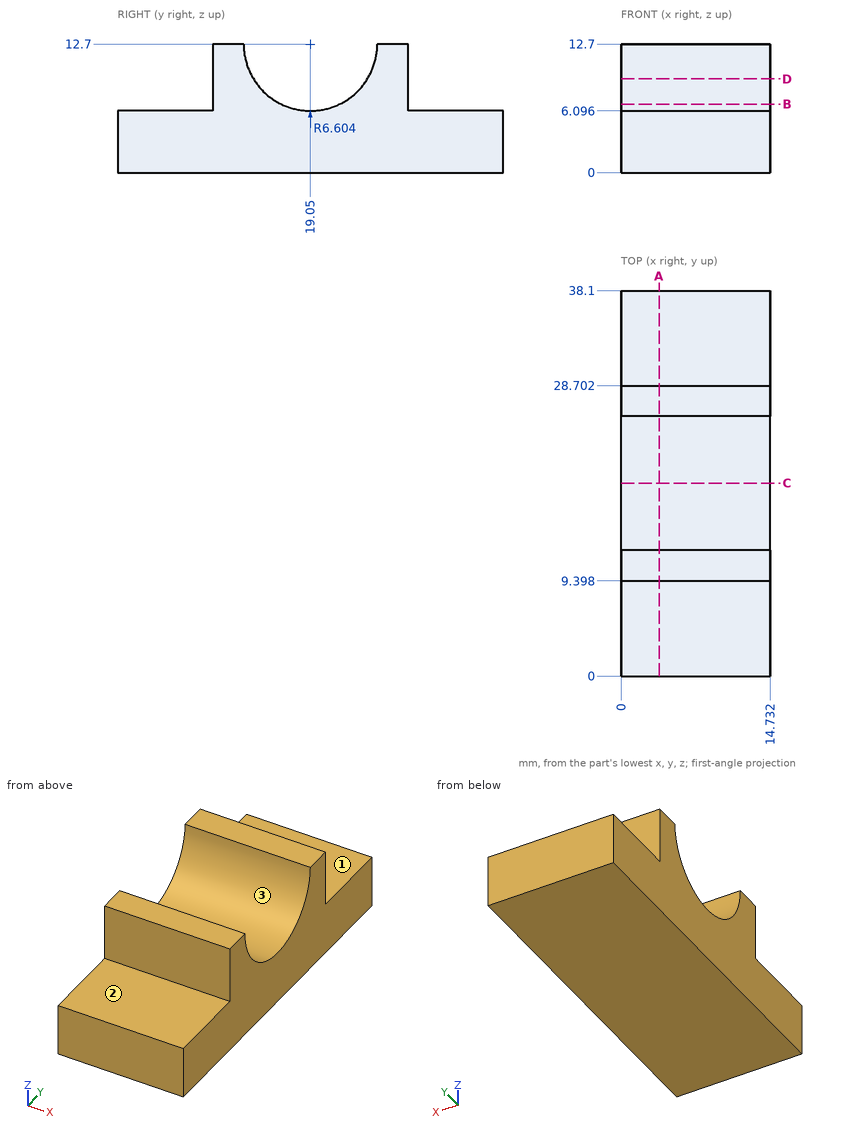
Geometry check sheet. Reference: drawing and pictorial views, mm from the part's lowest x, y, z. A direction names the side the tool comes from. Coordinates: 2 decimals unless noted, no trailing zeros. Order: outer loops, then holes, each group sorted by start corner. A loop starts at its lowest first (then second) coordinate and runs counter-clockwise, first axis right, second up. Notation, with made-up numbers: M 51,-26.5 L 56,-26.5 A24 ccw 56,-16.5 Z; hole C 34,-19 d9. An arc over 180 degrees is marked long. Return JSON: item names as keys, results as strings.
1) Access from +Z, -Z, +X, -X, +Y, -Y to the whole of each face (thin tool, end or side, straight path). Record for the marked faces 1, 2 and 3.
Answer list:
{"face 1": "+Z, +X, -X, +Y", "face 2": "+Z, +X, -X, -Y", "face 3": "+Z, +X, -X"}
2) Thickness scan on L1, parallel to Z at x = 13.5, y = 8; L2, parallel to Y at x = 9.75, z = 9.25; L3, parallel to Y at x = 13.25, z = 11.75. Record the ranges inside material, lowest first. Write a range as [from, to].
Answer list:
{"L1": "[0, 6.1]", "L2": "[9.4, 13.42], [24.68, 28.7]", "L3": "[9.4, 12.51], [25.59, 28.7]"}
3) Cross-section at D-D, the plane z = 9.25. Record the boundary of the cut face in (x, y).
Answer list:
{"outline": "M 0,9.4 L 14.73,9.4 L 14.73,13.42 L 0,13.42 Z; M 0,24.68 L 14.73,24.68 L 14.73,28.7 L 0,28.7 Z"}
4) Cross-section at A-A, the plane x = 3.75. Record the boundary of the cut face in (y, z), and give its area (3 significant figures).
Answer list:
{"outline": "M 0,0 L 38.1,0 L 38.1,6.1 L 28.7,6.1 L 28.7,12.7 L 25.65,12.7 A6.6 cw 12.45,12.7 L 9.4,12.7 L 9.4,6.1 L 0,6.1 Z", "area": "291 mm2"}
5) Cross-section at C-C, the plane y = 19.05. Record the boundary of the cut face in (x, z).
Answer list:
{"outline": "M 0,0 L 14.73,0 L 14.73,6.1 L 0,6.1 Z"}
6) Gauge pin test, flat ends, axial feed: pin 1 (3.5 mm diameter, centred on x = 5.5, z = 10, fed in from +Y); pin 2 (5 mm diameter, centred on x = 9, z = 5.5, fed in from -Y); pin 3 (5.5 mm diameter, centred on x = 7, z = 10.5, fed in from -Y); pin 4 (4.5 mm diameter, centred on x = 4.5, y = 35, fed in from +Z). Record the tip position at first contact, or that the pin passes through.
Answer list:
{"pin 1": "y = 28.7", "pin 2": "y = 0", "pin 3": "y = 9.4", "pin 4": "z = 6.1"}
7) Cross-section at B-B, the plane z = 6.75. Record the boundary of the cut face in (x, y).
Answer list:
{"outline": "M 0,9.4 L 14.73,9.4 L 14.73,16.18 L 0,16.18 Z; M 0,21.92 L 14.73,21.92 L 14.73,28.7 L 0,28.7 Z"}
